Design review of the part built by this model. Coordinates are the model's own, in mm. A direction names the side the tool comes from. Give positions to 0.01 mm unless a question says otherwise; leave off trailing zeros. Loops run counter-clockwise (first coordinate to the right, second up) from the corner with the lowest first, then second, coordinate; pieces in that order, holes last. Notation, with made-up numbers: (84, 73.5) -> (142, 73.5) arc R12 cw to (142, 95.5) -> close; hole circle Ø9 at (88, 62). An arc over 180 degrees is marked (long way). Use a Markdown table: item, result. Add a question column.
1. For pin 1 Ø2 at (y, z) = (-2, -19) entering from -X; pin 2 Ø5 at (x, y) = (-11, -6.5) entering from -Z; pin 3 Ø1.6 at (x, y) = (13, -11) entering from -Z, all flat-tipped, find the tip position at first contact; note any pin that passes through.
2. Add section A-A (z = -5.75). State the section outline as (x, y) points.
3. Draft analysis for pull direction X (two halves, no side actions). For faces 1 (the flat face through (-1, -15, -10)), 2 (the flat face through (-15, -7, -2)), 3 (the flat face through (17, -7, -13)), state which applies: pulls with the +X half, pulls with the -X half, needs draft (parallel to the pull), parting line crosses it, or undercut.
4. Add section C-C (y = -0.75). State the section outline as (x, z) points.
5. To check wall thickness, follow line 1 (X direction, y = -3.75, z = -5.25); line 2 (X direction, y = -6, z = -3.75); line 3 (X direction, y = -11.75, z = -9). State the ranges of each line that lie inside material, in increasing order.
6. For faces 4 (the flat face through (4.5, -8, -10)), 5 (the flat face through (-6, -7, -6)), 6 (the flat face through (16, -7, -8.5)), list the 3-axis set-ups (+Z, -Z, +X, -X, +Y, -Y) from which the entire face can be reached by the end or side of a thin tool; tool diameter is ignored.
```python
from build123d import *

# Parameters (mm, degrees)
F1_DEPTH = 15
F2_W     = 8.9
F2_H     = 11.8
F3_DEPTH = 25
F4_SIZE  = 0.3
F5_SIZE  = 0.5


with BuildPart() as f1:
    # F0 (on Front) → F1 (new body)
    with BuildSketch(Plane.XZ):
        with BuildLine():
            Line((6, 1), (-6, 1))
            Line((-6, 1), (-6, -3))
            ThreePointArc((-6, -3), (-6.75, -3.75), (-6, -4.5))
            Line((-6, -4.5), (-6, -5.7))
            Line((-6, -5.7), (-6, -7.7))
            ThreePointArc((-6, -7.7), (-6.8786796564, -9.8213203436), (-9, -10.7))
            Line((-9, -10.7), (-13, -10.7))
            ThreePointArc((-13, -10.7), (-15.1213203436, -9.8213203436), (-16, -7.7))
            Line((-16, -7.7), (-16, -5.7))
            Line((-16, -5.7), (-16, -3))
            Line((-16, -3), (-14.5, -3))
            Line((-14.5, -3), (-16, 0))
            Line((-16, 0), (-19, 0))
            Line((-19, 0), (-19, -7.7))
            ThreePointArc((-19, -7.7), (-17.2426406871, -11.9426406871), (-13, -13.7))
            Line((-13, -13.7), (-8.6602540378, -13.7))
            ThreePointArc((-8.6602540378, -13.7), (-3.6602540378, -15.0397459622), (0, -18.7))
            ThreePointArc((0, -18.7), (2.1961524227, -20.8961524227), (5.1961524227, -21.7))
            Line((5.1961524227, -21.7), (12, -21.7))
            ThreePointArc((12, -21.7), (15.5355339059, -20.2355339059), (17, -16.7))
            Line((17, -16.7), (17, -8.5))
            Line((17, -8.5), (14, -8.5))
            Line((14, -8.5), (12.5, -11.5))
            Line((12.5, -11.5), (14, -11.5))
            Line((14, -11.5), (14, -14.7))
            Line((14, -14.7), (14, -16.7))
            ThreePointArc((14, -16.7), (13.4142135624, -18.1142135624), (12, -18.7))
            Line((12, -18.7), (10, -18.7))
            ThreePointArc((10, -18.7), (7.1715728753, -17.5284271247), (6, -14.7))
            Line((6, -14.7), (6, -1))
            ThreePointArc((6, -1), (7, 0), (6, 1))
        make_face()
    extrude(amount=F1_DEPTH)

    # F2 (on face) → F3 (cut)
    with BuildSketch(Plane.XY.offset(1)):
        with Locations((0.05, -7.5)):
            Rectangle(F2_W, F2_H)
    extrude(amount=-F3_DEPTH, mode=Mode.SUBTRACT)

    # F4
    f4_edges = [f1.edges().sort_by_distance(p)[0] for p in [
        (11, -15, -18.7),
        (7.171573, -15, -17.528427),
        (6, -15, -7.85),
        (7, -15, 0),
        (0, -15, 1),
        (-6, -15, -1),
        (-6.75, -15, -3.75),
        (-6, -15, -6.1),
        (-6.87868, -15, -9.82132),
        (-11, -15, -10.7),
        (-15.12132, -15, -9.82132),
        (-16, -15, -5.35),
        (-15.25, -15, -3),
        (-15.25, -15, -1.5),
        (-17.5, -15, 0),
        (-19, -15, -3.85),
        (-17.242641, -15, -11.942641),
        (-10.830127, -15, -13.7),
        (-3.660254, -15, -15.039746),
        (2.196152, -15, -20.896152),
        (8.598076, -15, -21.7),
        (15.535534, -15, -20.235534),
        (17, -15, -12.6),
        (15.5, -15, -8.5),
        (13.25, -15, -10),
        (13.25, -15, -11.5),
        (14, -15, -14.1),
        (13.414214, -15, -18.114214),
        (11, 0, -18.7),
        (7.171573, 0, -17.528427),
        (6, 0, -7.85),
        (7, 0, 0),
        (0, 0, 1),
        (-6, 0, -1),
        (-6.75, 0, -3.75),
        (-6, 0, -6.1),
        (-6.87868, 0, -9.82132),
        (-11, 0, -10.7),
        (-15.12132, 0, -9.82132),
        (-16, 0, -5.35),
        (-15.25, 0, -3),
        (-15.25, 0, -1.5),
        (-17.5, 0, 0),
        (-19, 0, -3.85),
        (-17.242641, 0, -11.942641),
        (-10.830127, 0, -13.7),
        (-3.660254, 0, -15.039746),
        (2.196152, 0, -20.896152),
        (8.598076, 0, -21.7),
        (15.535534, 0, -20.235534),
        (17, 0, -12.6),
        (15.5, 0, -8.5),
        (13.25, 0, -10),
        (13.25, 0, -11.5),
        (14, 0, -14.1),
        (13.414214, 0, -18.114214),
    ]]
    chamfer(f4_edges, length=F4_SIZE)

    # F5
    f5_edges = [f1.edges().sort_by_distance(p)[0] for p in [
        (-4.4, -13.4, -6.826444),
        (4.5, -13.4, -10.329739),
        (4.5, -1.6, -10.329739),
        (-4.4, -1.6, -6.826444),
    ]]
    chamfer(f5_edges, length=F5_SIZE)


solid = f1.part
```
Taken from the geometry:
| question | item | result |
|---|---|---|
| 1 | pin 1 | stops at x = -0.39 |
| 1 | pin 2 | stops at z = -13.7 |
| 1 | pin 3 | stops at z = -21.7 |
| 2 | outline | (-19, -14.7) -> (-18.7, -15) -> (-16.3, -15) -> (-16, -14.7) -> (-16, -0.3) -> (-16.3, 0) -> (-18.7, 0) -> (-19, -0.3) -> close; (-6, -14.7) -> (-5.7, -15) -> (5.7, -15) -> (6, -14.7) -> (6, -0.3) -> (5.7, 0) -> (-5.7, 0) -> (-6, -0.3) -> close; hole (-4.4, -12.9) -> (-3.9, -13.4) -> (4, -13.4) -> (4.5, -12.9) -> (4.5, -2.1) -> (4, -1.6) -> (-3.9, -1.6) -> (-4.4, -2.1) -> close |
| 3 | face 1 | needs draft |
| 3 | face 2 | undercut |
| 3 | face 3 | pulls with the +X half |
| 4 | outline | (-19, -7.7) arc R6 ccw to (-13, -13.7) -> (-8.66, -13.7) arc R10 cw to (0, -18.7) arc R6 ccw to (5.2, -21.7) -> (12, -21.7) arc R5 ccw to (17, -16.7) -> (17, -8.5) -> (14, -8.5) -> (12.5, -11.5) -> (14, -11.5) -> (14, -16.7) arc R2 cw to (12, -18.7) -> (10, -18.7) arc R4 cw to (6, -14.7) -> (6, -1) arc R1 ccw to (6, 1) -> (-6, 1) -> (-6, -3) arc R0.75 ccw to (-6, -4.5) -> (-6, -7.7) arc R3 cw to (-9, -10.7) -> (-13, -10.7) arc R3 cw to (-16, -7.7) -> (-16, -3) -> (-14.5, -3) -> (-16, 0) -> (-19, 0) -> close |
| 5 | line 1 | x = -19 to -16, -6 to -4.4, 4.5 to 6 |
| 5 | line 2 | x = -19 to -16, -6.75 to -4.4, 4.5 to 6 |
| 5 | line 3 | x = -18.86 to -15.7, -6.3 to -4.4, 4.5 to 6, 13.75 to 17 |
| 6 | face 4 | +Z, -Z |
| 6 | face 5 | +Y, -Y |
| 6 | face 6 | +Z, +X, +Y, -Y |
